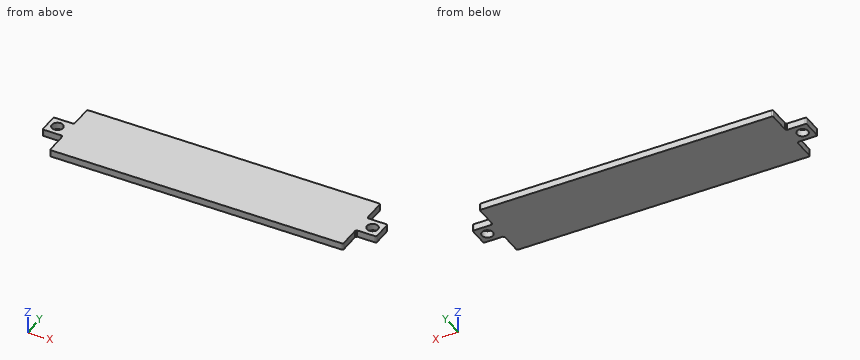
from build123d import *

# Parameters (mm, degrees)
F1_DEPTH = 2.032
F0_W     = 6.096
F0_H     = 6.096
F0_R     = 1.651
F2_DEPTH = 2.032
F3_DEPTH = 2.032
F4_R     = 0.381
F5_SIZE  = 0.381


with BuildPart() as f1:
    # F0 (on Top) → F1 (new body)
    with BuildSketch(Plane.XY):
        Polygon((-43.688, -10.1727), (43.688, -10.1727), (43.688, -3.175), (43.688, 2.921), (43.688, 10.1727), (-43.688, 10.1727), (-43.688, 3.048), (-43.688, -3.048), align=None)
    extrude(amount=F1_DEPTH)

    # F0 (on Top) → F2 (join)
    with BuildSketch(Plane.XY):
        with Locations((46.736, -0.127)):
            Rectangle(F0_W, F0_H)
        with Locations((46.99, -0.127)):
            Circle(F0_R, mode=Mode.SUBTRACT)
    extrude(amount=F2_DEPTH)

    # F0 (on Top) → F3 (join)
    with BuildSketch(Plane.XY):
        with Locations((-46.736, 0)):
            Rectangle(F0_W, F0_H)
        with Locations((-46.99, 0)):
            Circle(F0_R, mode=Mode.SUBTRACT)
    extrude(amount=F3_DEPTH)

    # F4
    f4_edges = [f1.edges().sort_by_distance(p)[0] for p in [
        (43.688, -10.1727, 1.016),
        (43.688, 10.1727, 1.016),
        (-43.688, -10.1727, 1.016),
        (-43.688, 10.1727, 1.016),
        (-49.784, 3.048, 1.016),
        (-49.784, -3.048, 1.016),
        (49.784, -3.175, 1.016),
        (49.784, 2.921, 1.016),
    ]]
    fillet(f4_edges, radius=F4_R)

    # F5
    f5_edges = [f1.edges().sort_by_distance(p)[0] for p in [
        (43.688, 2.921, 1.016),
        (43.688, -3.175, 1.016),
        (-43.688, -3.048, 1.016),
        (-43.688, 3.048, 1.016),
    ]]
    chamfer(f5_edges, length=F5_SIZE)


solid = f1.part
Could you check a few things on this model? Use its own coordinates, in mm. Give positions to 0.01 mm unless a question says otherwise; leave off trailing zeros. Order: outer loops, then holes, each group sorted by start corner. A loop starts at its lowest first (then second) coordinate and runs counter-clockwise, first axis right, second up. Notation, with made-up numbers: (21, 18) -> (53, 18) arc R28 ccw to (53, 46) -> close; hole circle Ø5 at (41.5, 50.5). An arc over 180 degrees is marked (long way). Return JSON: item names as keys, results as strings.
1. I need wall thicknesses on line 1 (Y direction, x = 46.99, z = 0.7) (3 decimals); line 2 (X direction, y = -1.5, z = 1); line 3 (Y direction, x = -46.99, z = 0.5). Which ranges of each line are inside material? Lowest first, please. Write a range as from..to.
Answer list:
{"line 1": "y = -3.175..-1.778, 1.524..2.921", "line 2": "x = -49.78..-47.68, -46.3..46.07, 47.91..49.78", "line 3": "y = -3.05..-1.65, 1.65..3.05"}
2. For pin 1 Ø1 at (x, z) = (-47, 1) entering from +Y; pin 2 Ø0.6 at (y, z) = (-5.5, 1) entering from +X; pin 3 Ø2 at (x, y) = (46.99, -0.127) entering from +Z; pin 4 Ø1 at (x, z) = (-45.5, 1) entering from -Y, each with a flat end and sliding along its axis, tell me the tip position at first contact or that it passes through.
Answer list:
{"pin 1": "stops at y = 3.05", "pin 2": "stops at x = 43.69", "pin 3": "passes through", "pin 4": "stops at y = -3.05"}
3. Imagine slicing it at B-B on z = 0.5. List the corners of the cut face in (x, y) for me (3 decimals).
Answer list:
{"outline": "(-49.784, -2.667) arc R0.381 ccw to (-49.403, -3.048) -> (-44.069, -3.048) -> (-43.688, -3.429) -> (-43.688, -9.792) arc R0.381 ccw to (-43.307, -10.173) -> (43.307, -10.173) arc R0.381 ccw to (43.688, -9.792) -> (43.688, -3.556) -> (44.069, -3.175) -> (49.403, -3.175) arc R0.381 ccw to (49.784, -2.794) -> (49.784, 2.54) arc R0.381 ccw to (49.403, 2.921) -> (44.069, 2.921) -> (43.688, 3.302) -> (43.688, 9.792) arc R0.381 ccw to (43.307, 10.173) -> (-43.307, 10.173) arc R0.381 ccw to (-43.688, 9.792) -> (-43.688, 3.429) -> (-44.069, 3.048) -> (-49.403, 3.048) arc R0.381 ccw to (-49.784, 2.667) -> close; hole circle Ø3.302 at (-46.99, 0); hole circle Ø3.302 at (46.99, -0.127)"}
4. Imagine slicing it at C-C on y = -5.5. List the corners of the cut face in (x, z) for me, then the cut area to 3 significant figures.
Answer list:
{"outline": "(-43.69, 0) -> (43.69, 0) -> (43.69, 2.03) -> (-43.69, 2.03) -> close", "area": "178 mm2"}
5. Imagine slicing it at A-A on x = -46.99. List the corners of the cut face in (y, z) for me, then the cut area to 3 significant figures.
Answer list:
{"outline": "(-3.05, 0) -> (-1.65, 0) -> (-1.65, 2.03) -> (-3.05, 2.03) -> close; (1.65, 0) -> (3.05, 0) -> (3.05, 2.03) -> (1.65, 2.03) -> close", "area": "5.68 mm2"}
